Design review of the part built by this model. Coordinates are the model's own, in mm. A direction names the side the tool comes from. Give positions to 0.01 mm unless a question says otherwise; leave off trailing zeros.
from build123d import *

# Parameters (mm, degrees)
F1_DEPTH = 29
F2_START = 25
F2_DEPTH = 4
F3_START = -25
F3_DEPTH = 4
F4_START = 26
F0_W     = 1.172746277
F0_H     = 3.0541475862
F0_H_2   = 0.957692816
F4_DEPTH = 2
F5_START = -26
F5_DEPTH = 2
F6_R     = 0.99999


# Not quite as in the source:
# - a fillet or chamfer is up to 0.001 mm smaller than in the source, because OpenCascade refuses the exact size


with BuildPart() as f1:
    # F0 (on Top) → F1 (new body, symmetric)
    with BuildSketch(Plane.XY):
        with BuildLine():
            Line((-4.0699890815, 24.2982581258), (-17.1110220253, 24.2982581258))
            ThreePointArc((-17.1110220253, 24.2982581258), (-17.7348526195, 23.6744275317), (-17.1110220253, 23.0505969375))
            Line((-17.1110220253, 23.0505969375), (-5.313185975, 22.8393822908))
            ThreePointArc((-5.313185975, 22.8393822908), (-4.3551853687, 22.085041739), (-5.313185975, 21.3307011873))
            Line((-5.313185975, 21.3307011873), (-17.3267684877, 21.0792534053))
            Line((-17.3267684877, 21.0792534053), (-17.7458468825, 20.7020826638))
            Line((-17.7458468825, 20.7020826638), (-17.3267684877, 20.2364402329))
            Line((-17.3267684877, 20.2364402329), (-5.313185975, 20.0213631141))
            ThreePointArc((-5.313185975, 20.0213631141), (-4.319986106, 19.2441805029), (-5.313185975, 18.4669978917))
            Line((-5.313185975, 18.4669978917), (-17.3407383263, 18.3133352548))
            Line((-17.3407383263, 18.3133352548), (-17.7458468825, 17.9431512952))
            Line((-17.7458468825, 17.9431512952), (-17.3407383263, 17.4823310226))
            Line((-17.3407383263, 17.4823310226), (-1.3890911359, 17.3372328281))
            ThreePointArc((-1.3890911359, 17.3372328281), (-0.492008259, 16.5730640292), (-1.3890911359, 15.8088952303))
            Line((-1.3890911359, 15.8088952303), (-17.3541552482, 15.6049273923))
            Line((-17.3541552482, 15.6049273923), (-17.7356619388, 15.1443993673))
            Line((-17.7356619388, 15.1443993673), (-17.5030883402, 14.7124780342))
            Line((-17.5030883402, 14.7124780342), (-1.3890911359, 14.5659030835))
            ThreePointArc((-1.3890911359, 14.5659030835), (-0.7437511811, 13.7670414267), (-1.3890911359, 12.9681797698))
            Line((-1.3890911359, 12.9681797698), (-17.4349947409, 12.6323343327))
            Line((-17.4349947409, 12.6323343327), (-17.7414808422, 12.3967602849))
            Line((-17.7414808422, 12.3967602849), (-17.5598803908, 11.9637120515))
            Line((-17.5598803908, 11.9637120515), (-1.3890911359, 11.5619925782))
            ThreePointArc((-1.3890911359, 11.5619925782), (-0.7146102661, 10.8705479652), (-1.3890911359, 10.1791033521))
            Line((-1.3890911359, 10.1791033521), (-17.4349947409, 9.7804863246))
            Line((-17.4349947409, 9.7804863246), (-17.57148467, 9.7804863246))
            Line((-17.57148467, 9.7804863246), (-17.7426468581, 9.5952115953))
            Line((-17.7426468581, 9.5952115953), (-17.5253339112, 9.1899503022))
            Line((-17.5253339112, 9.1899503022), (-1.3890911359, 8.7890890427))
            ThreePointArc((-1.3890911359, 8.7890890427), (-0.9606665076, 8.1417476758), (-1.3890911359, 7.494406309))
            Line((-1.3890911359, 7.494406309), (-17.5261050463, 7.0715243928))
            Line((-17.5261050463, 7.0715243928), (-17.7610386163, 6.8365903571))
            Line((-17.7610386163, 6.8365903571), (-17.5261050463, 6.3615223657))
            Line((-17.5261050463, 6.3615223657), (-1.3890911359, 5.9555862099))
            ThreePointArc((-1.3890911359, 5.9555862099), (-1.0583889027, 5.3565036505), (-1.3890911359, 4.7574210912))
            Line((-1.3890911359, 4.7574210912), (-17.4686410496, 4.3360450599))
            Line((-17.4686410496, 4.3360450599), (-17.8654273587, 3.982137423))
            Line((-17.8654273587, 3.982137423), (-17.4686410496, 3.5372773558))
            Line((-17.4686410496, 3.5372773558), (-1.7663730541, 3.1859290281))
            ThreePointArc((-1.7663730541, 3.1859290281), (-1.2007925503, 2.6075517307), (-1.7663730541, 2.0291744333))
            Line((-1.7663730541, 2.0291744333), (-17.4686410496, 1.6176853427))
            Line((-17.4686410496, 1.6176853427), (-17.7483521402, 1.1909720488))
            Line((-17.7483521402, 1.1909720488), (-17.4686410496, 0.8753370494))
            Line((-17.4686410496, 0.8753370494), (-1.7663730541, 0.4803371849))
            ThreePointArc((-1.7663730541, 0.4803371849), (-1.3259179646, -0.1754465338), (-1.7663730541, -0.8312302525))
            Line((-1.7663730541, -0.8312302525), (-17.5491847508, -1.244830048))
            ThreePointArc((-17.5491847508, -1.244830048), (-17.7110050083, -1.6010632209), (-17.5491847508, -1.9572963938))
            Line((-17.5491847508, -1.9572963938), (-1.9620249514, -2.3128963076))
            ThreePointArc((-1.9620249514, -2.3128963076), (-1.3537602225, -2.9351960402), (-1.9620249514, -3.5574957728))
            Line((-1.9620249514, -3.5574957728), (-17.5113877616, -3.9649778744))
            Line((-17.5113877616, -3.9649778744), (-17.7269522101, -4.4069844298))
            Line((-17.7269522101, -4.4069844298), (-17.312085256, -4.8613618128))
            Line((-17.312085256, -4.8613618128), (-2.2583589889, -5.0391620025))
            ThreePointArc((-2.2583589889, -5.0391620025), (-1.4871772278, -5.8195060119), (-2.2583589889, -6.5998500213))
            Line((-2.2583589889, -6.5998500213), (-17.5293660294, -6.7802165233))
            Line((-17.5293660294, -6.7802165233), (-17.7314169705, -7.1995011531))
            Line((-17.7314169705, -7.1995011531), (-17.3472613096, -7.6185795479))
            Line((-17.3472613096, -7.6185795479), (-3.3617539701, -7.9376399327))
            ThreePointArc((-3.3617539701, -7.9376399327), (-2.6814550827, -8.6336359286), (-3.3617539701, -9.3296319246))
            Line((-3.3617539701, -9.3296319246), (-17.4733772874, -9.5469430089))
            Line((-17.4733772874, -9.5469430089), (-17.710454762, -9.9222976714))
            Line((-17.710454762, -9.9222976714), (-17.335081473, -10.4161864147))
            Line((-17.335081473, -10.4161864147), (-3.228909336, -10.6137422845))
            Line((-3.228909336, -10.6137422845), (-1.7076556105, -10.1791201159))
            ThreePointArc((-1.7076556105, -10.1791201159), (-0.5341015375, -11.3842086866), (-1.7076556105, -12.5892972574))
            Line((-1.7076556105, -12.5892972574), (-3.189396346, -12.1941864491))
            Line((-3.189396346, -12.1941864491), (-17.2815993428, -12.3514840379))
            Line((-17.2815993428, -12.3514840379), (-17.7286379039, -12.7565935254))
            Line((-17.7286379039, -12.7565935254), (-17.3566557611, -13.1670760419))
            Line((-17.3566557611, -13.1670760419), (-3.5123708679, -13.3609642008))
            ThreePointArc((-3.5123708679, -13.3609642008), (-2.7387752862, -14.1454697919), (-3.5123708679, -14.929975383))
            Line((-3.5123708679, -14.929975383), (-17.3472613096, -15.1430249362))
            Line((-17.3472613096, -15.1430249362), (-17.6943112165, -15.5275696889))
            Line((-17.6943112165, -15.5275696889), (-17.3472613096, -15.9387048334))
            Line((-17.3472613096, -15.9387048334), (-2.1711152967, -16.1512456061))
            Line((-2.1711152967, -16.1512456061), (-2.1711152967, -19.0259180963))
            Line((-2.1711152967, -19.0259180963), (-1.1235726997, -19.0259180963))
            Line((-1.1235726997, -19.0259180963), (-1.1235726997, -15.1430249362))
            Line((-1.1235726997, -15.1430249362), (0.0491735773, -15.1430249362))
            Line((0.0491735773, -15.1430249362), (0.0491735773, -19.047325477))
            Line((0.0491735773, -19.047325477), (2.0417859778, -19.047325477))
            Line((2.0417859778, -19.047325477), (2.0417859778, 10.5479126796))
            Line((2.0417859778, 10.5479126796), (4.9630478024, 10.5479126796))
            Line((4.9630478024, 10.5479126796), (4.9630478024, 14.9210141972))
            Line((4.9630478024, 14.9210141972), (3.692939326, 14.901455239))
            Line((3.692939326, 14.901455239), (3.692939326, 11.8128489703))
            Line((3.692939326, 11.8128489703), (2.0417859778, 11.8128489703))
            Line((2.0417859778, 11.8128489703), (2.0417859778, 15.7654304057))
            ThreePointArc((2.0417859778, 15.7654304057), (2.3413387619, 16.4847297298), (3.0629034154, 16.7787838727))
            Line((3.0629034154, 16.7787838727), (13.6287314817, 16.7787838727))
            Line((13.6287314817, 16.7787838727), (13.9106530696, 16.9266853482))
            Line((13.9106530696, 16.9266853482), (13.9106530696, 17.7426013646))
            Line((13.9106530696, 17.7426013646), (2.7096215636, 17.9149005562))
            ThreePointArc((2.7096215636, 17.9149005562), (2.027143744, 18.6079572886), (2.7096215636, 19.301014021))
            Line((2.7096215636, 19.301014021), (13.7074142694, 19.4701869041))
            Line((13.7074142694, 19.4701869041), (13.7007343839, 19.9044408738))
            Line((13.7007343839, 19.9044408738), (2.7096215636, 20.0889185071))
            ThreePointArc((2.7096215636, 20.0889185071), (2.0410304994, 20.6815851852), (2.7096215636, 21.2742518634))
            Line((2.7096215636, 21.2742518634), (13.9556201175, 21.4712414891))
            Line((13.9556201175, 21.4712414891), (13.9486206756, 21.8708346796))
            Line((13.9486206756, 21.8708346796), (2.7096215636, 22.0614876598))
            ThreePointArc((2.7096215636, 22.0614876598), (2.0808096295, 22.7669365704), (2.7096215636, 23.472385481))
            Line((2.7096215636, 23.472385481), (13.9058372006, 23.6605741084))
            Line((13.9058372006, 23.6605741084), (13.8986392592, 24.088813075))
            Line((13.8986392592, 24.088813075), (13.6943962425, 24.271402508))
            Line((13.6943962425, 24.271402508), (0.4630363837, 24.271402508))
            ThreePointArc((0.4630363837, 24.271402508), (-0.6487056649, 23.3676230344), (-0.8640453452, 21.9511426985))
            Line((-0.8640453452, 21.9511426985), (-0.8640453452, 21.0152007639))
            ThreePointArc((-0.8640453452, 21.0152007639), (-0.7734316844, 19.7347502036), (-1.897772192, 19.1153772175))
            ThreePointArc((-1.897772192, 19.1153772175), (-2.6726628699, 19.513906378), (-3.0711919535, 20.2887970954))
            Line((-3.0711919535, 20.2887970954), (-2.680051839, 21.9092350453))
            ThreePointArc((-2.680051839, 21.9092350453), (-2.8952979424, 23.3828498722), (-4.0699890815, 24.2982581258))
        make_face()
    extrude(amount=F1_DEPTH, both=True)

    # F0 (on Top) → F2 (join)
    with BuildSketch(Plane.XY.offset(F2_START)):
        Polygon((0.0491735773, -21.6273944825), (0.0491735773, -19.047325477), (0.0491735773, -15.1430249362), (-1.1235726997, -15.1430249362), (-1.1235726997, -19.0259180963), (-1.1235726997, -21.6273944825), align=None)
    extrude(amount=F2_DEPTH)

    # F0 (on Top) → F3 (join)
    with BuildSketch(Plane.XY.offset(F3_START)):
        Polygon((0.0491735773, -21.6273944825), (0.0491735773, -19.047325477), (0.0491735773, -15.1430249362), (-1.1235726997, -15.1430249362), (-1.1235726997, -19.0259180963), (-1.1235726997, -21.6273944825), align=None)
    extrude(amount=-F3_DEPTH)

    # F0 (on Top) → F4 (join)
    with BuildSketch(Plane.XY.offset(F4_START)):
        with Locations((-0.5371995612, -23.1544682756)):
            Rectangle(F0_W, F0_H)
        with Locations((-0.5371995612, -25.1603884767)):
            Rectangle(F0_W, F0_H_2)
    extrude(amount=F4_DEPTH)

    # F0 (on Top) → F5 (join)
    with BuildSketch(Plane.XY.offset(F5_START)):
        with Locations((-0.5371995612, -23.1544682756)):
            Rectangle(F0_W, F0_H)
        with Locations((-0.5371995612, -25.1603884767)):
            Rectangle(F0_W, F0_H_2)
    extrude(amount=-F5_DEPTH)

    # F6 (radius 1 in the source; OpenCascade refuses exactly that, so slightly less here)
    f6_edges = [f1.edges().sort_by_distance(p)[0] for p in [
        (-0.5372, -25.639235, 28),
        (-0.5372, -25.639235, 26),
        (-0.5372, -25.639235, -26),
        (-0.5372, -25.639235, -28),
    ]]
    fillet(f6_edges, radius=F6_R)


solid = f1.part
Q1. Take a section at A-A (x = -12.5). Give the number of separate pieces and of enclosed holes in the cut face, plus the area to 3 significant figures.
Results:
separate pieces: 15
enclosed holes: 0
area: 869 mm2
Q2. Tool access review of faces 3 (the face through (-1.124, -22, 27)), 4 (the face through (2.042, 14, 0)), 5 (the face through (8, 16.779, 0)), 6 (the face through (1, -19.047, 0)): name each direction out of +Z, -Z, +X, -X, +Y, -Y from which nothing blocks a thin tool from reaching the whole face with its end or side.
Results:
face 3: +Z, -Z, -X, -Y
face 4: +Z, -Z
face 5: +Z, -Z, +X
face 6: +Z, -Z, +X, -Y
Q3. Draft analysis for pull direction Z (two halves, no side actions). For faces 1 (the face through (0.049, -17, 0)), 2 (the face through (-2.88, 23.36, 0.41)), state which applies: pulls with the +Z half, pulls with the -Z half, needs draft (parallel to the pull), parting line crosses it, or undercut.
Results:
face 1: undercut
face 2: needs draft
Q4. Wall thickness on line 1 (Y direction, x = 3, z = 12.5); line 2 (X direction, y = -17.5, z = 6); line 3 (Y direction, x = 0.5, z = 12.5): over which ranges is each line inside the solid? List them lowest first.
Results:
line 1: y = 10.55 to 11.81, 16.78 to 17.91, 19.31 to 20.08, 21.28 to 22.06, 23.48 to 24.27
line 2: x = -2.17 to -1.12, 0.05 to 2.04
line 3: y = -19.05 to 24.27
Q5. Insertion check: pin 1 (1.5 mm diameter, centred on x = -7, z = 17, fed in from -Y); pin 2 (8 mm diameter, centred on x = 1, z = 18, fed in from -Y); pin 3 (0.7 mm diameter, centred on y = 17.5, z = -13.5, fed in from +X). Each pin has a flat end and moves straight along its axis. Give the tip position at first contact, or say it passes through.
Results:
pin 1: stops at y = -16.09
pin 2: stops at y = -19.05
pin 3: stops at x = 13.91
